Geometry: see drawing. Coordinates: mm, zero at the bounding-box minimum. Coordinates: 2 decimals unless noted, no trailing zeros. Loops run counter-clockwise (first coordinate to the right, second up) from the corner with the lowest first, then second, coordinate; pieces in that order, holes last. Notation, with made-up numbers: (-26.5, 67) - (31.5, 67) arc R13 cw to (31.5, 79) - close; hole circle Ø9 at (50.5, 8.5). An arc over 180 degrees is marked (long way). Answer in a Markdown table with one row per item.
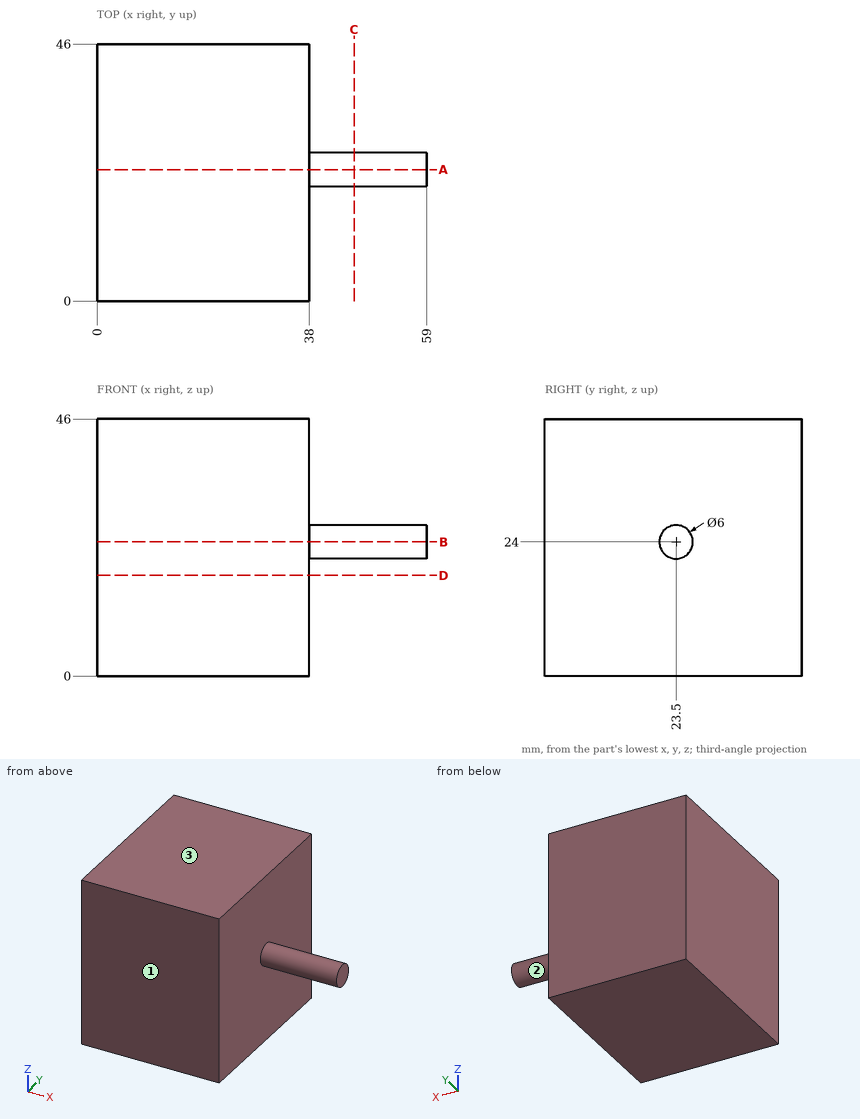
(1) First-contact query: pin 1 Ø10 at (x, z) = (52, 14) entering from +Y; pin 2 Ø3 at (y, z) = (30, 9.5) entering from +X; pin 3 Ø10 at (x, z) = (30, 9.5) entering from -Y. Flat tips, straight axial feed; report the tip coordinate or a pass-through.
Verdict:
| item | result |
|---|---|
| pin 1 | passes through |
| pin 2 | stops at x = 38 |
| pin 3 | stops at y = 0 |
(2) Pull-direction query (Z, two-part tool) for the marked faces 1, 2 and 3; classes: pulls with the +Z half, pulls with the -Z half, needs draft (parallel to the pull), parting line crosses it, or undercut.
Verdict:
| item | result |
|---|---|
| face 1 | needs draft |
| face 2 | parting line crosses it |
| face 3 | pulls with the +Z half |
(3) Cut plane B-B on z = 24. Output: boundary loops of the cut face in (x, y), then the cut area to 3 significant figures.
Verdict:
| item | result |
|---|---|
| outline | (0, 0) - (38, 0) - (38, 20.5) - (59, 20.5) - (59, 26.5) - (38, 26.5) - (38, 46) - (0, 46) - close |
| area | 1,870 mm² |
(4) Cut plane C-C on x = 46. Output: boundary loops of the cut face in (y, z).
Verdict:
| item | result |
|---|---|
| outline | circle Ø6 at (23.5, 24) |
(5) Cut plane A-A on y = 23.5. Output: boundary loops of the cut face in (x, z), then the cut area to 3 significant figures.
Verdict:
| item | result |
|---|---|
| outline | (0, 0) - (38, 0) - (38, 21) - (59, 21) - (59, 27) - (38, 27) - (38, 46) - (0, 46) - close |
| area | 1,870 mm² |
(6) Cut plane D-D on z = 18. Output: boundary loops of the cut face in (x, y), then the cut area to 3 significant figures.
Verdict:
| item | result |
|---|---|
| outline | (0, 0) - (38, 0) - (38, 46) - (0, 46) - close |
| area | 1,750 mm² |
(7) Ray query, probe 1 along X at (y, z) = (3.5, 10.5); probe 2 along Y at (x, z) = (40, 23); probe 3 along Y at (x, z) = (38.5, 22). Return the intervals inside material, ascending.
Verdict:
| item | result |
|---|---|
| probe 1 | x = 0 to 38 |
| probe 2 | y = 20.67 to 26.33 |
| probe 3 | y = 21.26 to 25.74 |
